Work out the finished part from the listing and answer in its coordinate system (mm). Coordinates: 2 decimals unless noted, no trailing zeros. Order: outer loops, then holes, each group sorted by start corner. A loop starts at its lowest first (then second) coordinate and runs counter-clockwise, first axis right, second up. Notation, with made-up numbers: M 63,8 L 112,8 A12 ccw 112,26 Z; hole C -30,-5.5 d4. An arc over 180 degrees is marked long. Answer in a Markdown table with one row per item. Add a question column.
Item 1: The part is cut by section A-A (y = 0). Write down the section's boundary in (x, z), then the cut area to 3 significant figures.
Item 2: The mould has two halves that part along X. Classify faces 1 (the face through (-2.8, 1.2, 0.5)), 2 (the face through (2.038, -0.045, 0.493)), 3 (the face through (-13, 0, 0)): released by +X, released by -X, zero draft, split by the parting line, or undercut.
Item 3: The part is cut by section D-D (y = 1.45). Write down the section's boundary in (x, z), then the cut area to 3 significant figures.
Item 4: A flat-ended cylindrical pin translates along its axis: pin 1 Ø1.6 at (x, y) = (0, 0) entering from -Z. Find the tip coordinate at first contact, or state that the pin passes through.
Item 5: The part is cut by section B-B (z = 0.55). Write down the section's boundary in (x, y).
Item 6: Consider line 1 (X direction, y = -0.65, z = 0.4); line 2 (X direction, y = -0.35, z = 0.6); line 3 (X direction, y = 1.75, z = 0.65). Determine where each line is inside the solid, lowest interval first. Write a range as from..to.
Item 7: The part is cut by section C-C (x = -0.5). Write down the section's boundary in (y, z), then the cut area to 3 significant figures.
from build123d import *

# Parameters (mm, degrees)
SKETCH1_R          = 1.01901554
EXTRUDE1_DEPTH     = 1
SKETCH2_R          = 1.6
CUT_EXTRUDE2_DEPTH = 28.366693334


with BuildPart() as part:
    # Sketch1 → Extrude1 (new body)
    with BuildSketch(Plane.XY):
        with BuildLine():
            Line((0, 2.038031079), (-25.234342, 2.038031079))
            ThreePointArc((-25.234342, 2.038031079), (-27.272373079, 0), (-25.234342, -2.038031079))
            Line((-25.234342, -2.038031079), (0, -2.038031079))
            ThreePointArc((0, -2.038031079), (2.038031079, 0), (0, 2.038031079))
        make_face()
        with Locations((-25.234342, 0)):
            Circle(SKETCH1_R, mode=Mode.SUBTRACT)
        Circle(SKETCH1_R, mode=Mode.SUBTRACT)
    extrude(amount=EXTRUDE1_DEPTH)

    # Sketch2 → Cut-Extrude2 (cut, through all)
    with BuildSketch(Plane.XY):
        with Locations((-2.8, 2.8)):
            Circle(SKETCH2_R)
    extrude(amount=CUT_EXTRUDE2_DEPTH, mode=Mode.SUBTRACT)


solid = part.part
Reply:
| question | item | result |
|---|---|---|
| 1 | outline | M -27.27,0 L -26.25,0 L -26.25,1 L -27.27,1 Z; M -24.22,0 L -1.02,0 L -1.02,1 L -24.22,1 Z; M 1.02,0 L 2.04,0 L 2.04,1 L 1.02,1 Z |
| 1 | area | 25.2 mm2 |
| 2 | face 1 | undercut |
| 2 | face 2 | released by +X |
| 2 | face 3 | zero draft |
| 3 | outline | M -26.67,0 L -3.66,0 L -3.66,1 L -26.67,1 Z; M -1.94,0 L 1.43,0 L 1.43,1 L -1.94,1 Z |
| 3 | area | 26.4 mm2 |
| 4 | pin 1 | passes through |
| 5 | outline | M -25.23,-2.04 L 0,-2.04 A2.04 ccw 0,2.04 L -1.39,2.04 A1.6 cw -4.21,2.04 L -25.23,2.04 A2.04 ccw Z; hole C -25.23,0 d2.04; hole C 0,0 d2.04 |
| 6 | line 1 | x = -27.17..-26.02, -24.45..-0.78, 0.78..1.93 |
| 6 | line 2 | x = -27.24..-26.19, -24.28..-0.96, 0.96..2.01 |
| 6 | line 3 | x = -26.28..-4.01, -1.59..1.04 |
| 7 | outline | M -2.04,0 L -0.89,0 L -0.89,1 L -2.04,1 Z; M 0.89,0 L 2.04,0 L 2.04,1 L 0.89,1 Z |
| 7 | area | 2.30 mm2 |
